```python
from build123d import *

# Parameters (mm, degrees)
F0_R     = 1.75
F1_DEPTH = 3
F2_R     = 3.25
F3_DEPTH = 1.5
F4_R     = 3
F5_R     = 1.25
F6_DEPTH = 3.001


with BuildPart() as f1:
    # F0 (on Top) → F1 (new body)
    with BuildSketch(Plane.XY):
        Polygon((43, 22.5), (0, 22.5), (-43, 22.5), (-43, 14.5), (-36, 14.5), (-36, 0), (-36, -14.5), (-43, -14.5), (-43, -22.5), (0, -22.5), (43, -22.5), (43, -14.5), (36, -14.5), (36, 0), (36, 14.5), (43, 14.5), align=None)
        with Locations((-39, -18.5)):
            Circle(F0_R, mode=Mode.SUBTRACT)
        with Locations((39, -18.5)):
            Circle(F0_R, mode=Mode.SUBTRACT)
        with Locations((-39, 18.5)):
            Circle(F0_R, mode=Mode.SUBTRACT)
        with Locations((39, 18.5)):
            Circle(F0_R, mode=Mode.SUBTRACT)
    extrude(amount=F1_DEPTH)

    # F2 (on face) → F3 (cut)
    with BuildSketch(Plane.XY.offset(3)):
        with Locations((-39, 18.5)):
            Circle(F2_R)
        with Locations((-39, -18.5)):
            Circle(F2_R)
        with Locations((39, 18.5)):
            Circle(F2_R)
        with Locations((39, -18.5)):
            Circle(F2_R)
    extrude(amount=-F3_DEPTH, mode=Mode.SUBTRACT)

    # F4
    f4_edges = [f1.edges().sort_by_distance(p)[0] for p in [
        (43, -22.5, 1.5),
        (43, -14.5, 1.5),
        (43, 14.5, 1.5),
        (43, 22.5, 1.5),
        (-43, -14.5, 1.5),
        (-43, -22.5, 1.5),
        (-43, 14.5, 1.5),
        (-43, 22.5, 1.5),
    ]]
    fillet(f4_edges, radius=F4_R)

    # F5 (on face) → F6 (cut, through all)
    with BuildSketch(Plane.XY.offset(3)):
        with Locations((-25, 15)):
            Circle(F5_R)
        with Locations((-20, 15)):
            Circle(F5_R)
        with Locations((-15, 15)):
            Circle(F5_R)
        with Locations((-10, 15)):
            Circle(F5_R)
        with Locations((-5, 15)):
            Circle(F5_R)
        with Locations((0, 15)):
            Circle(F5_R)
        with Locations((5, 15)):
            Circle(F5_R)
        with Locations((10, 15)):
            Circle(F5_R)
        with Locations((15, 15)):
            Circle(F5_R)
        with Locations((20, 15)):
            Circle(F5_R)
        with Locations((25, 15)):
            Circle(F5_R)
        with Locations((-25, 10)):
            Circle(F5_R)
        with Locations((-20, 10)):
            Circle(F5_R)
        with Locations((-15, 10)):
            Circle(F5_R)
        with Locations((-10, 10)):
            Circle(F5_R)
        with Locations((-5, 10)):
            Circle(F5_R)
        with Locations((0, 10)):
            Circle(F5_R)
        with Locations((5, 10)):
            Circle(F5_R)
        with Locations((10, 10)):
            Circle(F5_R)
        with Locations((15, 10)):
            Circle(F5_R)
        with Locations((20, 10)):
            Circle(F5_R)
        with Locations((25, 10)):
            Circle(F5_R)
        with Locations((-25, 5)):
            Circle(F5_R)
        with Locations((-20, 5)):
            Circle(F5_R)
        with Locations((-15, 5)):
            Circle(F5_R)
        with Locations((-10, 5)):
            Circle(F5_R)
        with Locations((-5, 5)):
            Circle(F5_R)
        with Locations((0, 5)):
            Circle(F5_R)
        with Locations((5, 5)):
            Circle(F5_R)
        with Locations((10, 5)):
            Circle(F5_R)
        with Locations((15, 5)):
            Circle(F5_R)
        with Locations((20, 5)):
            Circle(F5_R)
        with Locations((25, 5)):
            Circle(F5_R)
        with Locations((-25, 0)):
            Circle(F5_R)
        with Locations((-20, 0)):
            Circle(F5_R)
        with Locations((-15, 0)):
            Circle(F5_R)
        with Locations((-10, 0)):
            Circle(F5_R)
        with Locations((-5, 0)):
            Circle(F5_R)
        Circle(F5_R)
        with Locations((5, 0)):
            Circle(F5_R)
        with Locations((10, 0)):
            Circle(F5_R)
        with Locations((15, 0)):
            Circle(F5_R)
        with Locations((20, 0)):
            Circle(F5_R)
        with Locations((25, 0)):
            Circle(F5_R)
        with Locations((-25, -5)):
            Circle(F5_R)
        with Locations((-20, -5)):
            Circle(F5_R)
        with Locations((-15, -5)):
            Circle(F5_R)
        with Locations((-10, -5)):
            Circle(F5_R)
        with Locations((-5, -5)):
            Circle(F5_R)
        with Locations((0, -5)):
            Circle(F5_R)
        with Locations((5, -5)):
            Circle(F5_R)
        with Locations((10, -5)):
            Circle(F5_R)
        with Locations((15, -5)):
            Circle(F5_R)
        with Locations((20, -5)):
            Circle(F5_R)
        with Locations((25, -5)):
            Circle(F5_R)
        with Locations((-25, -10)):
            Circle(F5_R)
        with Locations((-20, -10)):
            Circle(F5_R)
        with Locations((-15, -10)):
            Circle(F5_R)
        with Locations((-10, -10)):
            Circle(F5_R)
        with Locations((-5, -10)):
            Circle(F5_R)
        with Locations((0, -10)):
            Circle(F5_R)
        with Locations((5, -10)):
            Circle(F5_R)
        with Locations((10, -10)):
            Circle(F5_R)
        with Locations((15, -10)):
            Circle(F5_R)
        with Locations((20, -10)):
            Circle(F5_R)
        with Locations((25, -10)):
            Circle(F5_R)
        with Locations((-25, -15)):
            Circle(F5_R)
        with Locations((-20, -15)):
            Circle(F5_R)
        with Locations((-15, -15)):
            Circle(F5_R)
        with Locations((-10, -15)):
            Circle(F5_R)
        with Locations((-5, -15)):
            Circle(F5_R)
        with Locations((0, -15)):
            Circle(F5_R)
        with Locations((5, -15)):
            Circle(F5_R)
        with Locations((10, -15)):
            Circle(F5_R)
        with Locations((15, -15)):
            Circle(F5_R)
        with Locations((20, -15)):
            Circle(F5_R)
        with Locations((25, -15)):
            Circle(F5_R)
    extrude(amount=-F6_DEPTH, mode=Mode.SUBTRACT)


solid = f1.part
```
Input: part model. Units: mm. Frame: model coordinates. A direction names the side the tool comes from. Coordinates: 2 decimals unless noted, no trailing zeros. Loops run counter-clockwise (first coordinate to the right, second up) from the corner with the lowest first, then second, coordinate; pieces in that order, holes last. Notation, with made-up numbers: M 19,76.25 L 25,76.25 A32 ccw 25,106.25 Z; hole C -32.5,-14.5 d3. An arc over 180 degrees is marked long. Use a Markdown table: item, result. Add a question column.
1) Line query: L1, parallel to Y at x = 38.5, z = 0.7; L2, parallel to X at y = 7.5, z = 2.75. Output: solid intervals per line, ascending. Write a range as from..to.
2) Set-up query: faces 1 (the cylindrical face through (-42.14, 15.4, 1.52)), 2 (the flat face through (38, -14.5, 1)), 3 (the cylindrical face through (14.73, -6.22, 1.52)), 4 (the flat face through (40.4, 17.1, 1.5)). Return all of +Z, -Z, +X, -X, +Y, -Y with unobstructed straight access to the full face (end or side cutting, diameter ignored); none if empty.
3) Draft query along Y for faces 5 (the cylindrical face through (21.155, 4.521, 1.521)), 6 (the cylindrical face through (42.1, 21.64, 1.52)), 7 (the cylindrical face through (-15.27, 3.78, 1.52)). Return one class per face: +Y half, -Y half, draft (parallel to the pull), parting line (faces both ways), or undercut.
4) Pin query (flat end, axial travel): P1, Ø4, axis at x = -31, y = -5.5, coming from the -Z side; P2, Ø4, axis at x = -39, y = -18.5, coming from the +Z side. Return the tip coordinate at first contact, or that it passes through.
5) Section B-B, the plane x = 10. Give the number of separate pieces and of enclosed holes in the cut face, plus the area to 3 significant figures.
6) Section A-A, the plane y = 18.5. Return the cut outline in (x, z), plus the area to 3 significant figures.
Answer below:
| question | item | result |
|---|---|---|
| 1 | L1 | -22.5..-20.18, -16.82..-14.5, 14.5..16.82, 20.18..22.5 |
| 1 | L2 | -36..36 |
| 2 | face 1 | +Z, -Z, -X |
| 2 | face 2 | +Z, -Z, +X |
| 2 | face 3 | +Z, -Z |
| 2 | face 4 | +Z |
| 3 | face 5 | undercut |
| 3 | face 6 | +Y half |
| 3 | face 7 | undercut |
| 4 | P1 | z = 0 |
| 4 | P2 | z = 1.5 |
| 5 | separate pieces | 8 |
| 5 | enclosed holes | 0 |
| 5 | area | 82.5 mm2 |
| 6 | outline | M -43,0 L -40.75,0 L -40.75,1.5 L -42.25,1.5 L -42.25,3 L -43,3 Z; M -37.25,0 L 37.25,0 L 37.25,1.5 L 35.75,1.5 L 35.75,3 L -35.75,3 L -35.75,1.5 L -37.25,1.5 Z; M 40.75,0 L 43,0 L 43,3 L 42.25,3 L 42.25,1.5 L 40.75,1.5 Z |
| 6 | area | 228 mm2 |
